Read the model definition and answer for the solid it produces. Units are mm, in the model's axes. Face numbers are marked on the shaded views. A direction names the side the tool comes from. Coordinates: 2 decimals unless noted, no trailing zeros. Loops run counter-clockwise (first coordinate to the right, second up) from the corner with the lowest first, then second, coordinate; pieces in that order, holes last. Notation, with made-up numbers: (-33.75, 47) -> (1.25, 47) arc R14 cw to (1.25, 66) -> close; hole circle Ø5 at (8.5, 26.5). An arc over 180 degrees is marked (long way). Answer as a JSON object with one key per item and string values. Group by question number.
Q1. For the marked faces 1, 2 and 3, determine the directions among +Z, -Z, +X, -X, +Y, -Y from which every point of the face is accessible in a straight line to the end or side of a thin tool.
Q2. The part is cut by section C-C on x = 96. Write down the section's boundary in (y, z), and give its area (3 significant figures).
Q3. The part is cut by section A-A on x = 45.5. Write down the section's boundary in (y, z).
Q4. The part is cut by section B-B on z = 0. Write down the section's boundary in (x, y), and give its area (3 significant figures).
Q5. Straight lines are drawn through the part: line 1 along Z through (x, y) = (96, 1.8); line 2 along Z through (x, y) = (31, 3); line 3 along Y through (x, z) = (41.5, -12.5). For each, find the intervals that lie inside material, in ascending order. Write a range as [from, to].
Q6. Each of these flat-tipped pins is pushed along its axis until it touches: P1, Ø1.5, axis at y = 9, z = 4.5, coming from the -X side; P2, Ø6.5, axis at x = 96, z = 0, coming from the -Y side; P3, Ø15, axis at x = 204, z = -6.5, coming from the -Y side; P4, Ø12, axis at y = 15.5, z = -0.5, coming from the -X side. Where does it stop, or does it pass through?
from build123d import *

# Parameters (mm, degrees)
EXTRUDE_1_DEPTH     = 15
CUT_EXTRUDE_1_DEPTH = 242.509337294
FILLET_1_R          = 8
SKETCH_4_R          = 3.5
CUT_EXTRUDE_2_DEPTH = 242.509337294
CUT_EXTRUDE_3_DEPTH = 242.979337961
FILLET_2_R          = 8


with BuildPart() as part:
    # 草圖2 → 填料-伸長1 (new, symmetric)
    with BuildSketch(Plane.XY):
        with BuildLine():
            Line((159.381107666, 13.248555109), (152.598076211, 1.5))
            ThreePointArc((152.598076211, 1.5), (151.5, 0.401923789), (150, 0))
            Line((150, 0), (0, 0))
            Line((0, 0), (0, 4.6))
            Line((0, 4.6), (147.344188762, 4.6))
            ThreePointArc((147.344188762, 4.6), (148.844188762, 5.001923789), (149.942264973, 6.1))
            Line((149.942264973, 6.1), (155.397390809, 15.548555109))
            Line((155.397390809, 15.548555109), (161.142860195, 25.5))
            ThreePointArc((161.142860195, 25.5), (162.240936407, 26.598076211), (163.740936407, 27))
            Line((163.740936407, 27), (240, 27))
            Line((240, 27), (240, 22.4))
            Line((240, 22.4), (166.396747645, 22.4))
            ThreePointArc((166.396747645, 22.4), (164.896747645, 21.998076211), (163.798671434, 20.9))
            Line((163.798671434, 20.9), (159.381107666, 13.248555109))
        make_face()
    extrude(amount=EXTRUDE_1_DEPTH, both=True)

    # 草圖3 → 除料-伸長1 (cut, through all)
    with BuildSketch(Plane(origin=(0, 4.6, 0), x_dir=(1, 0, 0), z_dir=(0, 1, 0))):
        with BuildLine():
            Line((33.076655966, 2.5), (58.923344034, 2.5))
            ThreePointArc((58.923344034, 2.5), (64.25, 0), (58.923344034, -2.5))
            Line((58.923344034, -2.5), (33.076655966, -2.5))
            ThreePointArc((33.076655966, -2.5), (27.75, 0), (33.076655966, 2.5))
        make_face()
    extrude(amount=-CUT_EXTRUDE_1_DEPTH, mode=Mode.SUBTRACT)

    # 圓角1
    fillet_1_edges = [part.edges().sort_by_distance(p)[0] for p in [
        (240, 24.7, -15),
        (240, 24.7, 15),
    ]]
    fillet(fillet_1_edges, radius=FILLET_1_R)

    # 草圖4 → 除料-伸長2 (cut, through all)
    with BuildSketch(Plane(origin=(0, 4.6, 0), x_dir=(1, 0, 0), z_dir=(0, 1, 0))):
        with Locations(Location((96, 0, 0), (0, 0, 180))):
            Circle(SKETCH_4_R)
    extrude(amount=-CUT_EXTRUDE_2_DEPTH, mode=Mode.SUBTRACT)

    # 草圖5 → 除料-伸長3 (cut, through all)
    with BuildSketch(Plane(origin=(0, 27, 0), x_dir=(1, 0, 0), z_dir=(0, 1, 0))):
        with BuildLine():
            Line((174, -2.5), (215, -2.5))
            ThreePointArc((215, -2.5), (217.5, 0), (215, 2.5))
            Line((215, 2.5), (174, 2.5))
            ThreePointArc((174, 2.5), (171.5, 0), (174, -2.5))
        make_face()
    extrude(amount=-CUT_EXTRUDE_3_DEPTH, mode=Mode.SUBTRACT)

    # 圓角2
    fillet_2_edges = [part.edges().sort_by_distance(p)[0] for p in [
        (0, 2.3, -15),
        (0, 2.3, 15),
    ]]
    fillet(fillet_2_edges, radius=FILLET_2_R)


solid = part.part
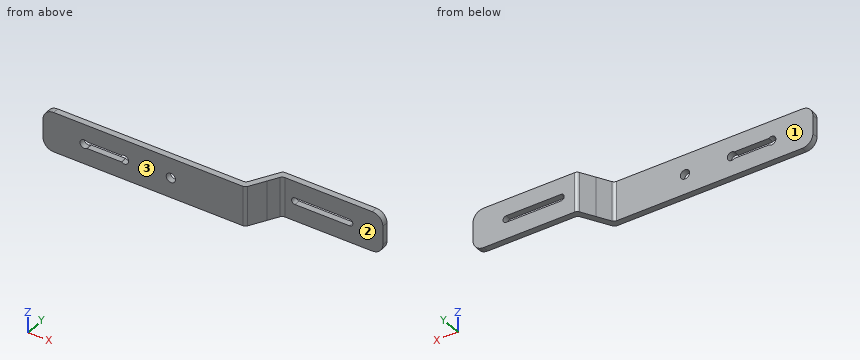
Final values:
{
 "1": {"face 1": "+Z, -Z, -X, +Y", "face 2": "+Z, -Z, +X, -Y", "face 3": "+Z, -Z, +X, -X, -Y"},
 "2": {"outline": "(0, -15) -> (4.6, -15) -> (4.6, -3.5) -> (0, -3.5) -> close; (0, 3.5) -> (4.6, 3.5) -> (4.6, 15) -> (0, 15) -> close", "area": "106 mm2"},
 "3": {"outline": "(0, -15) -> (4.6, -15) -> (4.6, -2.5) -> (0, -2.5) -> close; (0, 2.5) -> (4.6, 2.5) -> (4.6, 15) -> (0, 15) -> close"},
 "4": {"outline": "(0, 0) -> (27.75, 0) -> (27.75, 4.6) -> (0, 4.6) -> close; (64.25, 0) -> (92.5, 0) -> (92.5, 4.6) -> (64.25, 4.6) -> close; (99.5, 0) -> (150, 0) arc R3 ccw to (152.6, 1.5) -> (163.8, 20.9) arc R3 cw to (166.4, 22.4) -> (171.5, 22.4) -> (171.5, 27) -> (163.74, 27) arc R3 ccw to (161.14, 25.5) -> (149.94, 6.1) arc R3 cw to (147.34, 4.6) -> (99.5, 4.6) -> close; (217.5, 22.4) -> (240, 22.4) -> (240, 27) -> (217.5, 27) -> close", "area": "752 mm2"},
 "5": {"line 1": "z = [-15, -3.5], [3.5, 15]", "line 2": "z = [-15, -3.25], [3.25, 15]", "line 3": "y = [0, 4.6]"},
 "6": {"P1": "stops at x = 151.18", "P2": "passes through", "P3": "stops at y = 22.4", "P4": "stops at x = 151.91"}
}
